Part model, mm, in its own coordinate system. Face numbers are marked on the shaded views. Give positions to 0.01 mm unless a question says otherwise; leave off trailing zeros. Loops run counter-clockwise (first coordinate to the right, second up) from the corner with the lowest first, then second, coordinate; pieces in that order, holes last. Notation, with made-up numbers: M 6,11.25 L 28,11.25 A13 ccw 28,18.25 Z; hole C -12,-10.75 d7. An arc over 180 degrees is marked long. Put each result on its own line as item: value. Start each with the question number.
```python
from build123d import *

# Parameters (mm, degrees)
EXTRUDE_1_DEPTH   = 2
EXTRUDE_2_DEPTH   = 5
HOLE_WIZARD_M21_D = 2.4


with BuildPart() as part:
    # Эскиз1 → Бобышка-Вытянуть1 (new body)
    with BuildSketch(Plane(origin=(0, 0, 0), x_dir=(1, 0, 0), z_dir=(0, 1, 0))):
        with BuildLine():
            ThreePointArc((0, 0), (-25, 3.980394669), (-50, 0))
            Line((-50, 0), (-50, 5.4))
            ThreePointArc((-50, 5.4), (-25, 9.13662189), (0, 5.4))
            Line((0, 5.4), (0, 0))
        make_face()
    extrude(amount=EXTRUDE_1_DEPTH)

    # Эскиз1<3> → Бобышка-Вытянуть2 (add)
    with BuildSketch(Plane(origin=(0, 0, 0), x_dir=(1, 0, 0), z_dir=(0, 1, 0))):
        with BuildLine():
            Line((-50, -2.106904802), (-50, 0))
            ThreePointArc((-50, 0), (-25, 3.980394669), (0, 0))
            Line((0, 0), (0, -2.106904802))
            ThreePointArc((0, -2.106904802), (-25, 1.980394669), (-50, -2.106904802))
        make_face()
    extrude(amount=EXTRUDE_2_DEPTH)

    # Отверстие с зазором M21 (through all)
    with Locations(Plane(origin=(0, 0, 0), x_dir=(-1, 0, 0), z_dir=(0, -1, 0))):
        with Locations((42.5, 4.770770064), (25, 6.63662189), (7.5, 4.770770064)):
            Hole(HOLE_WIZARD_M21_D / 2)


solid = part.part
```
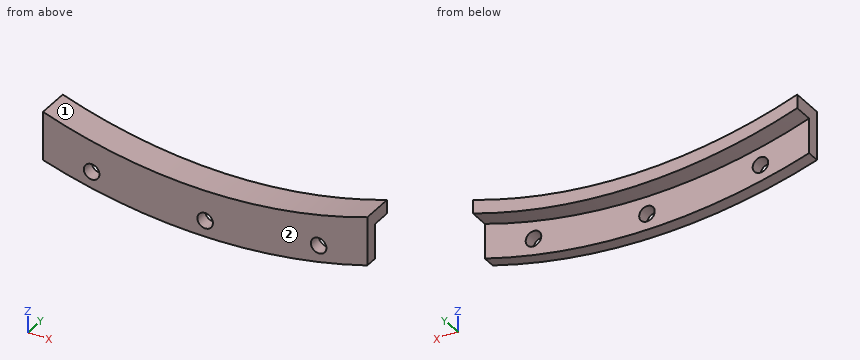
1) Band-saw the part on D-D on x = -7.5. Give the cut face in (y, z), then the cut area to 3 significant figures.
2) Wall check: L1, parallel to X at y = 1.3, z = -5; L2, parallel to Z at x = -7.5, y = 0.4; L3, parallel to Y at x = -28.5, z = -7.25. Give the ranges that are in metal, low to high.
3) Mould opens along X. For the marked faces 1 and 2 say: +X half, -X half, draft (parallel to the pull), parting line (faces both ways), or undercut.
4) Band-saw the part on B-B on z = 1. Give the cut face in (x, y).
5) Pin check, flat tips, straight feed: pin 1 Ø1.5 at (x, z) = (-23, 0) entering from +Y; pin 2 Ø4 at (x, z) = (-25, -6.64) entering from -Y; pin 3 Ø3 at (x, z) = (-7.5, -4.77) entering from +Y; pin 4 Ø1.5 at (x, y) = (-37, 2.5) entering from -Z. Stop position of each tip, or through.
6) Band-saw the part on A-A on x = -25. Give the cut face in (y, z).
7) Band-saw the part on C-C on y = 0.8. Give the cut face in (x, z).
Evaluation:
1. outline: M 0,-7.33 L 2,-7.33 L 2,-5.97 L 0,-5.97 Z; M 0,-3.57 L 2,-3.57 L 2,-2.06 L 5,-2.06 L 5,0 L 0,0 Z
1. area: 16.0 mm2
2. L1: -50 to -43.68, -41.32 to -8.68, -6.32 to 0
2. L2: -7.33 to -5.97, -3.57 to 0
2. L3: 0 to 2
3. face 1: undercut
3. face 2: draft
4. outline: M -50,0 L -46.43,0 L -46.43,5 L -50,5 Z; M -3.57,0 L 0,0 L 0,5 L -3.57,5 Z
5. pin 1: through
5. pin 2: y = 0
5. pin 3: y = 2
5. pin 4: z = -8.37
6. outline: M 0,-9.14 L 2,-9.14 L 2,-7.84 L 0,-7.84 Z; M 0,-5.44 L 2,-5.44 L 2,-3.98 L 5,-3.98 L 5,-1.98 L 0,-1.98 Z
7. outline: M -50,-5.4 A85.5 ccw 0,-5.4 L 0,2.11 A78.5 cw -50,2.11 Z; hole C -42.5,-4.77 d2.4; hole C -25,-6.64 d2.4; hole C -7.5,-4.77 d2.4
